Geometry: see drawing. Coordinates: mm, zero at the bounding-box minimum. A direction names the side the tool comes from. Give positions to 0.01 mm unless a question says otherwise; leave off trailing zeros. Write each loop counter-clockwise with the first axis right and the second up, starting at its lowest first coordinate (ties: lowest second). Pieces come first, ordered by that corner, then holes. Notation, with made-up numbers: (75, 53.25) - (82, 53.25) arc R11 ccw to (82, 57.25) - close; hole circle Ø2 at (64.25, -10). An arc over 180 degrees is marked (long way). Answer as CSV lines item,"result". Start each with the question number.
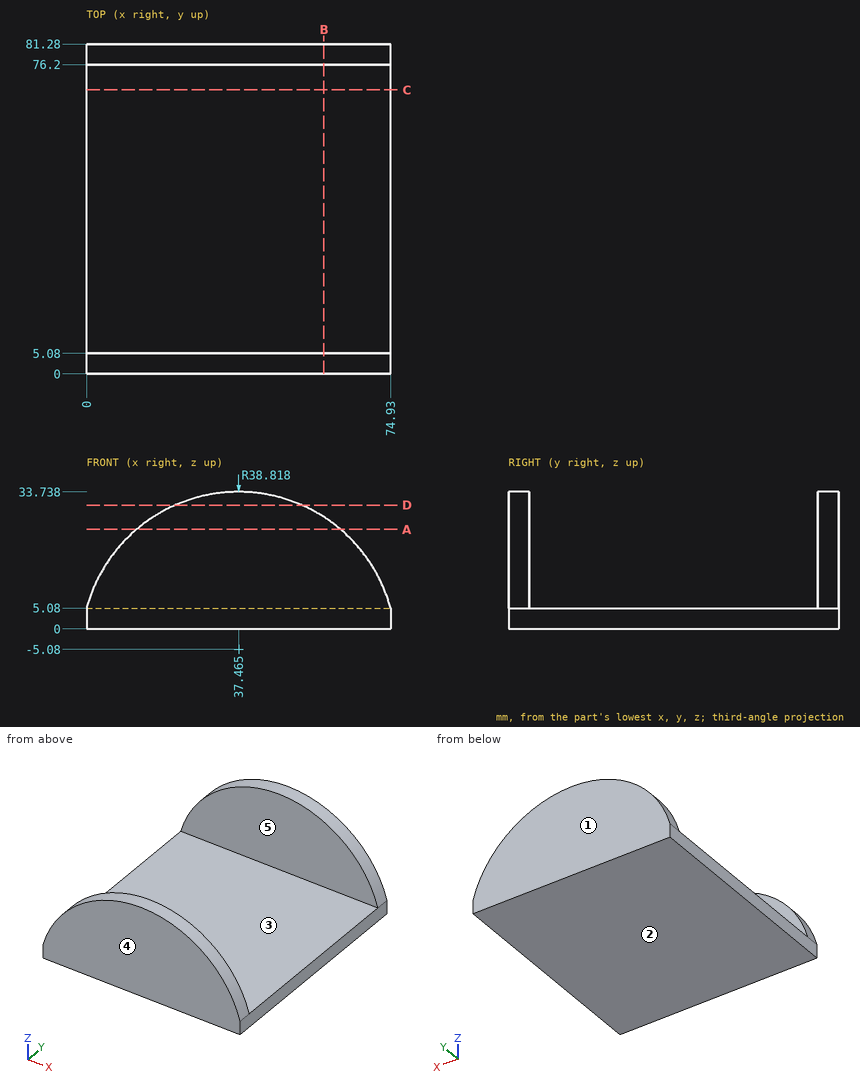
1) Cut plane B-B on x = 58.5. Output: boundary loops of the cut face in (y, z) (1 decimal), and give its area (3 significant figures).
2) Cut plane D-D on z = 30.5. Output: boundary loops of the cut face in (x, y), and give its area (3 significant figures).
3) Contact query for a flat-ended pin moving along its axis: P1, Ø5, axis at x = 34.5, y = 49, coming from the +Z side. Output: stop coordinate, or through.
4) Reachability of the marked faces 4 and 5 from +Z, -Z, +X, -X, +Y, -Y: full face, straight path, thin tool, end or side. Return the list, or none.
5) Cut plane A-A on z = 24.5. Output: boundary loops of the cut face in (x, y), and give its area (3 significant figures).
6) Pull-direction query (Y, two-part tool) for the marked faces 1, 2 and 3; classes: +Y half, -Y half, draft (parallel to the pull), parting line (faces both ways), or undercut.
7) Material intervals for line 1 (Y direction, x = 39.5, z = 9); line 2 (Z direction, x = 25, y = 42.5), sorted ascending. Write a range as from..to.
8) Cut plane C-C on y = 70. Output: boundary loops of the cut face in (x, z), and give its area (3 significant figures).
Numbers:
1,outline,"(0, 0) - (81.3, 0) - (81.3, 27.5) - (76.2, 27.5) - (76.2, 5.1) - (5.1, 5.1) - (5.1, 27.5) - (0, 27.5) - close"
1,area,"641 mm²"
2,outline,"(21.94, 0) - (52.99, 0) - (52.99, 5.08) - (21.94, 5.08) - close; (21.94, 76.2) - (52.99, 76.2) - (52.99, 81.28) - (21.94, 81.28) - close"
2,area,"315 mm²"
3,P1,"stops at z = 5.08"
4,face 4,"+Z, -Z, +X, -X, -Y"
4,face 5,"+Z, +X, -X"
5,outline,"(12.33, 0) - (62.6, 0) - (62.6, 5.08) - (12.33, 5.08) - close; (12.33, 76.2) - (62.6, 76.2) - (62.6, 81.28) - (12.33, 81.28) - close"
5,area,"511 mm²"
6,face 1,"+Y half"
6,face 2,"draft"
6,face 3,"undercut"
7,line 1,"y = 0..5.08, 76.2..81.28"
7,line 2,"z = 0..5.08"
8,outline,"(0, 0) - (74.93, 0) - (74.93, 5.08) - (0, 5.08) - close"
8,area,"381 mm²"
